The model under review builds one solid part; all positions refer to its coordinate system, in mm. Coordinates: 2 decimals unless noted, no trailing zeros. Order: outer loops, then holes, each group sorted by start corner. A loop starts at its lowest first (then second) coordinate and runs counter-clockwise, first axis right, second up.
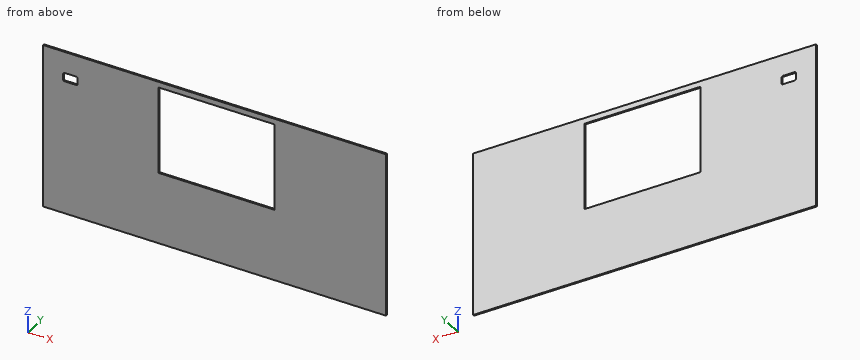
```python
from build123d import *

# Parameters (mm, degrees)
SKETCH1_W           = 1190
SKETCH1_H           = 576
BOSS_EXTRUDE1_DEPTH = 5
SKETCH2_R           = 1.5
CUT_EXTRUDE1_DEPTH  = 10
SKETCH3_W           = 150
SKETCH3_H           = 150
CUT_EXTRUDE2_DEPTH  = 10
SKETCH4_W           = 402
SKETCH4_H           = 305
CUT_EXTRUDE3_DEPTH  = 6
CUT_EXTRUDE4_DEPTH  = 10


with BuildPart() as part:
    # Sketch1 → Boss-Extrude1 (new body)
    with BuildSketch(Plane(origin=(0, 0, 0), x_dir=(1, 0, 0), z_dir=(0, 1, 0))):
        Rectangle(SKETCH1_W, SKETCH1_H)
    extrude(amount=BOSS_EXTRUDE1_DEPTH)

    # Sketch2 → Cut-Extrude1 (cut)
    with BuildSketch(Plane(origin=(595, 0, 0), x_dir=(0, 0, -1), z_dir=(1, 0, 0))):
        with Locations((-278, 2.5)):
            Circle(SKETCH2_R)
        with Locations(Location((278, 2.5, 0), (0, 0, 180))):
            Circle(SKETCH2_R)
    cut_extrude1 = extrude(amount=-CUT_EXTRUDE1_DEPTH, mode=Mode.SUBTRACT)

    # Mirror1: Cut-Extrude1 across plane
    add(cut_extrude1.mirror(Plane(origin=(0, 0, 0), x_dir=(0, 0, 1), z_dir=(1, 0, 0))), mode=Mode.SUBTRACT)

    # Sketch3 → Cut-Extrude2 (cut)
    with BuildSketch(Plane(origin=(0, 5, 0), x_dir=(1, 0, 0), z_dir=(0, 1, 0))):
        with Locations((5, -143)):
            Rectangle(SKETCH3_W, SKETCH3_H)
    extrude(amount=-CUT_EXTRUDE2_DEPTH, mode=Mode.SUBTRACT)

    # Sketch4 → Cut-Extrude3 (cut)
    with BuildSketch(Plane(origin=(0, 5, 0), x_dir=(1, 0, 0), z_dir=(0, 1, 0))):
        with Locations((7, -115.5)):
            Rectangle(SKETCH4_W, SKETCH4_H)
    extrude(amount=-CUT_EXTRUDE3_DEPTH, mode=Mode.SUBTRACT)

    # Sketch5 → Cut-Extrude4 (cut)
    with BuildSketch(Plane(origin=(0, 5, 0), x_dir=(1, 0, 0), z_dir=(0, 1, 0))):
        with BuildLine():
            Line((-520, -183), (-480, -183))
            ThreePointArc((-480, -183), (-476.464466094, -184.464466094), (-475, -188))
            Line((-475, -188), (-475, -208))
            ThreePointArc((-475, -208), (-476.464466094, -211.535533906), (-480, -213))
            Line((-480, -213), (-520, -213))
            ThreePointArc((-520, -213), (-523.535533906, -211.535533906), (-525, -208))
            Line((-525, -208), (-525, -188))
            ThreePointArc((-525, -188), (-523.535533906, -184.464466094), (-520, -183))
        make_face()
    extrude(amount=-CUT_EXTRUDE4_DEPTH, mode=Mode.SUBTRACT)


solid = part.part
```
(1) We need section B-B, the plane z = 66.5. Write out the cut boundary in (x, y), and give its area (3 significant figures).
A:
outline: (-595, 0) - (-194, 0) - (-194, 5) - (-595, 5) - close; (208, 0) - (595, 0) - (595, 5) - (208, 5) - close
area: 3,940 mm2
(2) For pin 1 Ø1.8 at (y, z) = (2.5, 278) entering from +X; pin 2 Ø2.5 at (y, z) = (2.5, -278) entering from -X, all flat-tipped, find the tip position at first contact; note any pin that passes through.
A:
pin 1: stops at x = 585
pin 2: stops at x = -585
(3) We need section C-C, the plane y = 2.5. Count the separate pieces of the cut face and the enclosed holes in it, and give its area (3 significant figures).
A:
separate pieces: 1
enclosed holes: 2
area: 561,000 mm2
(4) Wall thickness on probe 1 along Y at (x, z) = (-588, 278); probe 2 along Z at (x, y) = (169, 2.5); probe 3 along X at (y, z) = (3.35, 248): over which ranges is each line inside the solid? List them lowest first.
A:
probe 1: y = 0 to 1, 4 to 5
probe 2: z = -288 to -37, 268 to 288
probe 3: x = -595 to -194, 208 to 595
(5) We need section A-A, the plane x = -134. Write out the cut boundary in (y, z), and give its area (4 significant figures).
A:
outline: (0, -288) - (5, -288) - (5, -37) - (0, -37) - close; (0, 268) - (5, 268) - (5, 288) - (0, 288) - close
area: 1,355 mm2
